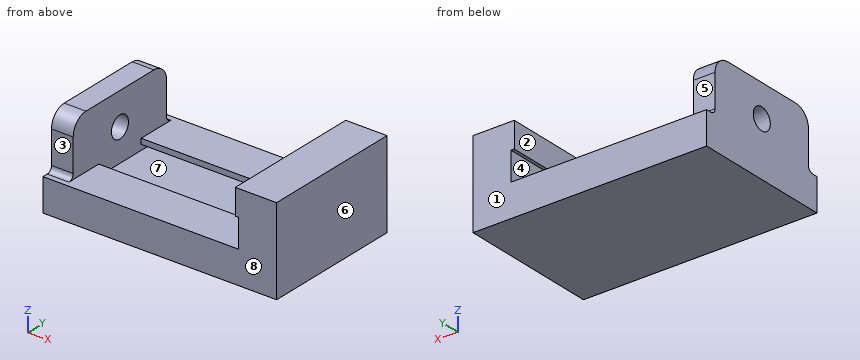
Autodesk Fusion 360 part; units mm, degrees
sketch "Sketch1" plane through (0, 0, 0) normal (0, 1, 0) x (1, 0, 0)
  line L0 (0, 0) -> (215, 0)
  line L1 (215, 0) -> (215, -30)
  line L2 (215, -30) -> (0, -30)
  line L3 (0, -30) -> (0, 0)
  line L4 (215, 0) -> (180, 0)
  line L5 (180, 0) -> (180, -80)
  line L6 (180, -80) -> (215, -80)
  line L7 (215, -80) -> (215, 0)
  line L8 (180, -80) -> (177, -80)
  line L9 (177, -80) -> (177, -56.3222)
  line L10 (177, -56.3222) -> (180, -56.3222)
  line L11 (180, -56.3222) -> (180, -80)
  dimension "d1" = 215
  dimension "d2" = 30
  dimension "d3" = 35
  dimension "d4" = 80
  dimension "d21" = 3
  dimension "d22" = 23.6778
extrude "Extrude1" add sketch "Sketch1" along normal blind 130 contours L0 L2 L3 L5 | L0 L1 L2 L4 L5 L7 | L2 L5 L6 L7 L11
sketch "Sketch2" plane through (0, 0, 0) normal (-1, 0, 0) x (0, -1, 0)
  line L0 (0, 0) -> (0, 30)
  line L1 (0, 30) -> (-130, 30)
  line L2 (-130, 30) -> (-130, 0)
  line L3 (-130, 0) -> (0, 0)
  line L4 (-10, 35) -> (-10, 65)
  line L5 (-25, 80) -> (-105, 80)
  line L6 (-120, 65) -> (-120, 35)
  line L7 (0, 80) -> (-130, 80)
  arc A0 (-105, 80) -> (-120, 65) centre (-105, 65) ccw
  arc A1 (-10, 65) -> (-25, 80) centre (-25, 65) ccw
  line L8 (-130, 30) -> (-125, 30)
  line L9 (-5, 30) -> (0, 30)
  arc A2 (-125, 30) -> (-120, 35) centre (-125, 35) ccw
  arc A3 (-10, 35) -> (-5, 30) centre (-5, 35) ccw
  circle A4 centre (-65, 50) radius 10
  line L10 (-105, 20) -> (-25, 20)
  line L11 (-105, 20) -> (-90, 25)
  line L12 (-40, 25) -> (-25, 20)
  line L13 (-90, 25) -> (-90, 30)
  line L14 (-40, 25) -> (-40, 30)
  point P0 (-10, 80)
  point P1 (-120, 80)
  dimension "d7" = 110
  dimension "d8" = 15
  dimension "d9" = 5
  dimension "d10" = 20
  dimension "d13" = 80
  dimension "d14" = 5
  dimension "d15" = 5
  dimension "d16" = 25
  dimension "d17" = 50
extrude "Extrude2" add sketch "Sketch2" against normal blind 20 contours L1 L4 L5 L6 L7 A0 A1 A2 A3
extrude "Extrude3" cut sketch "Sketch2" against normal up to surface (160 mm away) from surface at -20 contours L1 L10 L11 L12 L13 L14
extrude "Extrude4" add sketch "Sketch1" along normal blind 130 contours L5 L8 L9 L10 L11
Design review of the part built by this model. Coordinates are the model's own, in mm. Face numbers are marked on the shaded views. A direction names the side the tool comes from. Coordinates: 2 decimals unless noted, no trailing zeros. Loops run counter-clockwise (first coordinate to the right, second up) from the corner with the lowest first, then second, coordinate; pieces in that order, holes last. Notation, with made-up numbers: (-16.5, 39) - (4.5, 39) arc R25 cw to (4.5, 68) - close; hole circle Ø3 at (17.25, 24). An arc over 180 degrees is marked (long way). Use CSV: the item, a comma, the result in double quotes. Start each with the question number.
1) Consider section A-A on y = 65. Write out the cut boundary in (x, z).
2) Consider section B-B on z = 50. Write out the cut boundary in (x, y).
3) Wall thickness on L1, parallel to X at y = 16.5, z = 44; L2, parallel to Z at x = 5, y = 65; L3, parallel to X at y = 96.5, z = 74.5: over which ranges is each line inside the solid? List them lowest first. Write a range as from..to.
4) Tool access review of the marked faces 1, 2, 3 and 4: name each direction out of +Z, -Z, +X, -X, +Y, -Y from which nothing blocks a thin tool from reaching the whole face with its end or side.
5) Consider section D-D on x = 135.5. Write out the cut boundary in (y, z).
6) For pin 1 Ø6 at (x, y) = (48, 80.5) entering from +Z; pin 2 Ø10 at (x, z) = (14, 46.5) entering from +Y; pin 3 Ø10 at (x, z) = (14, 45.5) entering from -Y, all flat-tipped, find the tip position at first contact; note any pin that passes through.
7) The part is to be moulded in two halves that separate along Y. For the marked faces 5, 6, 7 and 8, say which applies: +Y half, -Y half, draft (parallel to the pull), parting line (faces both ways), or undercut.
8) Consider section C-C on z = 71. Write out the cut boundary in (x, y).
Geometry says:
1,outline,"(0, 0) - (215, 0) - (215, 80) - (177, 80) - (177, 56.32) - (180, 56.32) - (180, 20) - (20, 20) - (20, 40) - (0, 40) - close; (0, 60) - (20, 60) - (20, 80) - (0, 80) - close"
2,outline,"(0, 10) - (20, 10) - (20, 55) - (0, 55) - close; (0, 75) - (20, 75) - (20, 120) - (0, 120) - close; (180, 0) - (215, 0) - (215, 130) - (180, 130) - close"
3,L1,"0..20, 180..215"
3,L2,"0..40, 60..80"
3,L3,"0..20, 177..215"
4,face 1,"+Z, -Z, +X, -X, +Y"
4,face 2,"+Z, +Y, -Y"
4,face 3,"+Z, -X, -Y"
4,face 4,"none"
5,outline,"(0, 0) - (130, 0) - (130, 30) - (90, 30) - (90, 25) - (105, 20) - (25, 20) - (40, 25) - (40, 30) - (0, 30) - close"
6,pin 1,"z = 20"
6,pin 2,"y = 120"
6,pin 3,"y = 10"
7,face 5,"+Y half"
7,face 6,"draft"
7,face 7,"undercut"
7,face 8,"-Y half"
8,outline,"(0, 11.25) - (20, 11.25) - (20, 118.75) - (0, 118.75) - close; (177, 0) - (215, 0) - (215, 130) - (177, 130) - close"
